```python
from build123d import *

# Parameters (mm, degrees)
SKETCH_1_R           = 2.85
EXTRUDE_1_DEPTH      = 31.5
SKETCH_3_W           = 5.9
SKETCH_3_H           = 5.9
EXTRUDE_2_DEPTH      = 5
SKETCH_4_R           = 5
EXTRUDE_3_DEPTH      = 7
SKETCH_6_R           = 11.5
EXTRUDE_4_DEPTH      = 2
SKETCH_8_R           = 4.5
CUT_EXTRUDE_2_DEPTH  = 7.5
SKETCH_9_R           = 1.25
CUT_EXTRUDE_3_DEPTH  = 5.5
SKETCH_10_R          = 1.175
CUT_EXTRUDE_7_DEPTH  = 10
SKETCH_12_W          = 5.9
SKETCH_12_H          = 5.9
EXTRUDE_5_DEPTH      = 45
SKETCH_15_W          = 5.9
SKETCH_15_H          = 20.04910328
EXTRUDE_6_DEPTH      = 6
SKETCH_16_R          = 1.175
CUT_EXTRUDE_8_DEPTH  = 10
SKETCH_18_W          = 41.5
SKETCH_18_H          = 3.1
CUT_EXTRUDE_9_DEPTH  = 10
SKETCH_19_W          = 46.016613228
SKETCH_19_H          = 26.924390235
CUT_EXTRUDE_10_DEPTH = 10
SKETCH_21_OUTSIDE_W  = 37.01
SKETCH_21_OUTSIDE_H  = 37.01
SKETCH_21_OUTSIDE_R  = 2.85
CUT_EXTRUDE_11_DEPTH = 10
SKETCH_22_R          = 1.6
CUT_EXTRUDE_12_DEPTH = 3


with BuildPart() as part:
    # 스케치1 → 보스-돌출1 (new body)
    with BuildSketch(Plane.XY):
        Circle(SKETCH_1_R)
    extrude(amount=EXTRUDE_1_DEPTH)

    # 스케치3 → 보스-돌출2 (add)
    with BuildSketch(Plane(origin=(0, 0, 0), x_dir=(-1, 0, 0), z_dir=(0, 0, -1))):
        Rectangle(SKETCH_3_W, SKETCH_3_H)
    extrude(amount=EXTRUDE_2_DEPTH)

    # 스케치4 → 보스-돌출3 (add)
    with BuildSketch(Plane(origin=(0, 0, -5), x_dir=(-1, 0, 0), z_dir=(0, 0, -1))):
        Circle(SKETCH_4_R)
    extrude(amount=EXTRUDE_3_DEPTH)

    # 스케치6 → 보스-돌출4 (add)
    with BuildSketch(Plane(origin=(0, 0, -12), x_dir=(-1, 0, 0), z_dir=(0, 0, -1))):
        Circle(SKETCH_6_R)
    extrude(amount=EXTRUDE_4_DEPTH)

    # 스케치8 → 컷-돌출2 (cut)
    with BuildSketch(Plane(origin=(0, 0, -14), x_dir=(-1, 0, 0), z_dir=(0, 0, -1))):
        Circle(SKETCH_8_R)
    extrude(amount=-CUT_EXTRUDE_2_DEPTH, mode=Mode.SUBTRACT)

    # 스케치9 → 컷-돌출3 (cut)
    with BuildSketch(Plane(origin=(0, 0, -14), x_dir=(-1, 0, 0), z_dir=(0, 0, -1))):
        with Locations((3.444150891, 8.314915793)):
            Circle(SKETCH_9_R)
        with Locations((-3.444150891, 8.314915793)):
            Circle(SKETCH_9_R)
        with Locations((8.314915793, 3.444150891)):
            Circle(SKETCH_9_R)
        with Locations((8.314915793, -3.444150891)):
            Circle(SKETCH_9_R)
        with Locations((3.444150891, -8.314915793)):
            Circle(SKETCH_9_R)
        with Locations((-3.444150891, -8.314915793)):
            Circle(SKETCH_9_R)
        with Locations((-8.314915793, -3.444150891)):
            Circle(SKETCH_9_R)
        with Locations((-8.314915793, 3.444150891)):
            Circle(SKETCH_9_R)
    extrude(amount=-CUT_EXTRUDE_3_DEPTH, mode=Mode.SUBTRACT)

    # 스케치10 → 컷-돌출7 (cut)
    with BuildSketch(Plane(origin=(0, 2.95, 0), x_dir=(1, 0, 0), z_dir=(0, 1, 0))):
        with Locations(Location((0, 2.2, 0), (0, 0, 180))):
            Circle(SKETCH_10_R)
    extrude(amount=-CUT_EXTRUDE_7_DEPTH, mode=Mode.SUBTRACT)

    # 스케치12 → 보스-돌출5 (add)
    with BuildSketch(Plane.XY.offset(31.5)):
        Rectangle(SKETCH_12_W, SKETCH_12_H)
    extrude(amount=EXTRUDE_5_DEPTH)

    # 스케치15 → 보스-돌출6 (add)
    with BuildSketch(Plane.XY.offset(76.5)):
        Rectangle(SKETCH_15_W, SKETCH_15_H)
    extrude(amount=EXTRUDE_6_DEPTH)

    # 스케치16 → 컷-돌출8 (cut)
    with BuildSketch(Plane(origin=(0, 2.95, 0), x_dir=(1, 0, 0), z_dir=(0, 1, 0))):
        with Locations(Location((0, -33.7, 0), (0, 0, 270))):
            Circle(SKETCH_16_R)
    extrude(amount=-CUT_EXTRUDE_8_DEPTH, mode=Mode.SUBTRACT)

    # 스케치18 → 컷-돌출9 (cut)
    with BuildSketch(Plane(origin=(2.95, 0, 0), x_dir=(0, 0, -1), z_dir=(1, 0, 0))):
        with Locations((-15.75, -1.4)):
            Rectangle(SKETCH_18_W, SKETCH_18_H)
    extrude(amount=-CUT_EXTRUDE_9_DEPTH, mode=Mode.SUBTRACT)

    # 스케치19 → 컷-돌출10 (cut)
    with BuildSketch(Plane(origin=(2.95, 0, 0), x_dir=(0, 0, -1), z_dir=(1, 0, 0))):
        with Locations((-59.491693386, -3.437643478)):
            Rectangle(SKETCH_19_W, SKETCH_19_H)
    extrude(amount=-CUT_EXTRUDE_10_DEPTH, mode=Mode.SUBTRACT)

    # 스케치21 outside → 컷-돌출11 (cut)
    with BuildSketch(Plane.XY.offset(36.483386772)):
        Rectangle(SKETCH_21_OUTSIDE_W, SKETCH_21_OUTSIDE_H)
        Circle(SKETCH_21_OUTSIDE_R, mode=Mode.SUBTRACT)
    extrude(amount=-CUT_EXTRUDE_11_DEPTH, mode=Mode.SUBTRACT)

    # 스케치22 → 컷-돌출12 (cut)
    with BuildSketch(Plane(origin=(0, 2.95, 0), x_dir=(1, 0, 0), z_dir=(0, 1, 0))):
        with Locations(Location((0, -5, 0), (0, 0, 180))):
            Circle(SKETCH_22_R)
    extrude(amount=-CUT_EXTRUDE_12_DEPTH, mode=Mode.SUBTRACT)


solid = part.part
```
Read the model definition and answer for the solid it produces. Units are mm, in the model's axes. A direction names the side the tool comes from. Give positions to 0.01 mm unless a question says otherwise; leave off trailing zeros. Write each loop counter-clockwise with the first axis right and the second up, starting at its lowest first coordinate (ties: lowest second). Pieces come first, ordered by that corner, then holes. Notation, with made-up numbers: (51, -25.75) -> (60, -25.75) arc R16 cw to (60, 1.25) -> close; hole circle Ø3 at (13.5, 86.5). An arc over 180 degrees is marked (long way). Answer in a Markdown table with one row per item.
1) Section D-D on x = 3.75 is taken. Give the vertices of the cut face in (y, z).
Results list:
| item | result |
|---|---|
| outline | (-10.87, -14) -> (-9.53, -14) -> (-9.53, -12) -> (-10.87, -12) -> close; (-7.1, -14) -> (-2.49, -14) -> (-2.49, -6.5) -> (2.49, -6.5) -> (2.49, -14) -> (7.1, -14) -> (7.1, -12) -> (3.31, -12) -> (3.31, -5) -> (-3.31, -5) -> (-3.31, -12) -> (-7.1, -12) -> close; (9.53, -14) -> (10.87, -14) -> (10.87, -12) -> (9.53, -12) -> close |
2) A tool of negligible diameter and unlimited length cuts with its end or side. For faces 5 (the cylindrical face through (0.59, 4.46, -10.3)), 6 (the flat face through (0, 0.15, 16)), 7 (the flat face through (-5, -2, -12)), from which of +Z, -Z, +X, -X, +Y, -Y can it reach the whole face along a straight path? Write none if from no direction.
Results list:
| item | result |
|---|---|
| face 5 | -Z |
| face 6 | +Z, +X, -X, -Y |
| face 7 | +Z |
3) Section A-A on x = 0 is taken. Count the separate pieces of the cut face and the enclosed holes in it, plus the area to 3 significant figures.
Results list:
| item | result |
|---|---|
| separate pieces | 4 |
| enclosed holes | 0 |
| area | 139 mm^2 |
4) Section B-B on z = -2.2 is taken. Give the vertices of the cut face in (x, y) (3 decimals).
Results list:
| item | result |
|---|---|
| outline | (-2.95, 0.15) -> (-1.175, 0.15) -> (-1.175, 2.95) -> (-2.95, 2.95) -> close; (1.175, 0.15) -> (2.95, 0.15) -> (2.95, 2.95) -> (1.175, 2.95) -> close |
5) Each of these flat-tipped pins is pushed along its axis until it touches: pin 1 Ø1 at (x, y) = (8.5, -7) entering from +Z; pin 2 Ø5 at (y, z) = (-0.5, 9) entering from +X; pin 3 Ø4.5 at (x, z) = (1.5, 18) entering from -Y. Where does it stop, or does it pass through?
Results list:
| item | result |
|---|---|
| pin 1 | z = -12 |
| pin 2 | x = 2.85 |
| pin 3 | y = 0.15 |
6) Straight lines are drawn through the part: line 1 (Z direction, x = 0.5, y = 2); line 2 (Z direction, x = 0, y = 1) (3 decimals); line 3 (Z direction, x = -2, y = -4.75). For each, find the intervals that lie inside material, in ascending order. Write a range as [from, to].
Results list:
| item | result |
|---|---|
| line 1 | [-6.5, -3.26], [-1.14, 3.48], [6.52, 32.64], [34.76, 36.48] |
| line 2 | [-6.5, -3.375], [-1.025, 3.4], [6.6, 32.525], [34.875, 36.483] |
| line 3 | [-14, -12] |
7) Determine the mould class of faces 1 (the flat face through (-5, 0, -14)), 2 (the cylindrical face through (-7.394, -2.599, -13.014)), 3 (the cylindrical face through (-3.281, -7.076, -13.014)), 4 (the cylindrical face through (1.5, 11.4, -13)) for opening direction Y: released by +Y, released by -Y, zero draft, split by the parting line, or undercut.
Results list:
| item | result |
|---|---|
| face 1 | zero draft |
| face 2 | undercut |
| face 3 | undercut |
| face 4 | split by the parting line |
8) Section C-C on y = 4 is taken. Give the vertices of the cut face in (x, z), plus the area to 3 significant figures.
Results list:
| item | result |
|---|---|
| outline | (-10.78, -14) -> (-9.43, -14) -> (-9.43, -12) -> (-10.78, -12) -> close; (-7.2, -14) -> (-2.06, -14) -> (-2.06, -6.5) -> (2.06, -6.5) -> (2.06, -14) -> (7.2, -14) -> (7.2, -12) -> (3, -12) -> (3, -5) -> (-3, -5) -> (-3, -12) -> (-7.2, -12) -> close; (9.43, -14) -> (10.78, -14) -> (10.78, -12) -> (9.43, -12) -> close |
| area | 45.2 mm^2 |
